from build123d import *

# Parameters (mm, degrees)
F0_R     = 4.838468
F0_W     = 33.466397
F0_H     = 30.935322
F0_R_2   = 5.460503
F1_DEPTH = 5.08


with BuildPart() as f1:
    # F0 (on Top) → F1 (new body)
    with BuildSketch(Plane.XY):
        with BuildLine():
            ThreePointArc((17.891966, -1.952547), (32.435058, 11.67451), (37.801563, 30.868229))
            ThreePointArc((37.801563, 30.868229), (-18.093211, 62.692563), (-16.933151, -1.616599))
            Line((-16.933151, -1.616599), (17.891966, -1.952547))
        make_face()
        with Locations((-12.703, 51.397717)):
            Circle(F0_R, mode=Mode.SUBTRACT)
        with Locations((1.265535, 25.170104)):
            Rectangle(F0_W, F0_H, mode=Mode.SUBTRACT)
        with Locations((13.170184, 51.397717)):
            Circle(F0_R_2, mode=Mode.SUBTRACT)
        with BuildLine():
            ThreePointArc((-10.608257, -4.338439), (-13.834146, -3.124943), (-16.933151, -1.616599))
            Line((-16.933151, -1.616599), (-16.933151, -58.892032))
            Line((-16.933151, -58.892032), (-16.933151, -60.651779))
            Line((-16.933151, -60.651779), (17.891966, -60.651779))
            Line((17.891966, -60.651779), (17.891966, -1.952547))
            ThreePointArc((17.891966, -1.952547), (15.052123, -3.282136), (12.109917, -4.366543))
            Line((12.109917, -4.366543), (12.109917, -56.126706))
            Line((12.109917, -56.126706), (-10.608257, -56.126706))
            Line((-10.608257, -56.126706), (-10.608257, -50.480825))
            Line((-10.608257, -50.480825), (-10.608257, -4.338439))
        make_face()
        with BuildLine():
            Line((17.891966, -1.952547), (-16.933151, -1.616599))
            ThreePointArc((-16.933151, -1.616599), (-13.834146, -3.124943), (-10.608257, -4.338439))
            ThreePointArc((-10.608257, -4.338439), (-7.87319, -5.109583), (-5.087015, -5.668589))
            ThreePointArc((-5.087015, -5.668589), (0.33248, -6.136051), (5.761954, -5.804015))
            ThreePointArc((5.761954, -5.804015), (8.967599, -5.225107), (12.109917, -4.366543))
            ThreePointArc((12.109917, -4.366543), (15.052123, -3.282136), (17.891966, -1.952547))
        make_face()
        with BuildLine():
            ThreePointArc((5.761954, -5.804015), (0.33248, -6.136051), (-5.087015, -5.668589))
            Line((-5.087015, -5.668589), (-5.087015, -50.480825))
            Line((-5.087015, -50.480825), (5.761954, -50.64771))
            Line((5.761954, -50.64771), (5.761954, -5.804015))
        make_face()
    extrude(amount=F1_DEPTH)


solid = f1.part
Work out the finished part from the listing and answer in its coordinate system (mm). A direction names the side the tool comes from. Give positions to 0.01 mm unless a question says otherwise; leave off trailing zeros. Loops run counter-clockwise (first coordinate to the right, second up) from the corner with the lowest first, then second, coordinate; pieces in that order, holes last. Notation, with made-up numbers: (8, 89.25) -> (36, 89.25) arc R17 cw to (36, 118.25) -> close; hole circle Ø2 at (14, 39.5). An arc over 180 degrees is marked (long way). Use a Markdown table: item, result. Add a question column.
1. Determine the mould class of faces 3 (the flat face through (17.892, -32, 3)), 4 (the flat face through (0, -60.652, 3)), 5 (the cylindrical face through (-13.3, 56.2, 2.5)) for opening direction Y: released by +Y, released by -Y, zero draft, split by the parting line, or undercut.
2. For faces 1 (the flat face through (-15.468, 25, 3)), 2 (the flat face through (0, 5, 5.08)), determine the directions among +Z, -Z, +X, -X, +Y, -Y from which every point of the face is accessible in a straight line to the end or side of a thin tool.
3. Find the intervals of material crossed by probe 1 along X at (y, z) = (-19, 4.15); probe 2 along X at (y, z) = (55.5, 0.4); probe 3 along Y at (x, z) = (2.5, 4.7), in increasing order.
4. Section D-D on y = 16 is taken. Determine the outline of the cut face in (x, z).
5. Section C-C on z = 1.95 is taken. Determine the outline of the cut face in (x, y), and give its area (3 significant figures).
6. Section A-A on y = -12 is taken. Determine the outline of the cut face in (x, z).
7. Section B-B on x = -13.5 is taken. Determine the outline of the cut face in (y, z).
8. Flat-ended cylindrical pins translate along their axes: pin 1 Ø1.5 at (x, z) = (-1.5, 4) entering from +Y; pin 2 Ø1.5 at (y, z) = (-29.5, 3.5) entering from -X; pin 3 Ø1.5 at (y, z) = (-27.5, 2) entering from +X. Find the tip coordinate at first contact, or state that the pin passes through.
Results below:
| question | item | result |
|---|---|---|
| 1 | face 3 | zero draft |
| 1 | face 4 | released by -Y |
| 1 | face 5 | undercut |
| 2 | face 1 | +Z, -Z |
| 2 | face 2 | +Z, +X, -X, +Y, -Y |
| 3 | probe 1 | x = -16.93 to -10.61, -5.09 to 5.76, 12.11 to 17.89 |
| 3 | probe 2 | x = -26.82 to -15.27, -10.14 to 9.57, 16.77 to 28.41 |
| 3 | probe 3 | y = -60.65 to -56.13, -50.6 to 9.7, 40.64 to 67.84 |
| 4 | outline | (-33.09, 0) -> (-15.47, 0) -> (-15.47, 5.08) -> (-33.09, 5.08) -> close; (18, 0) -> (34.68, 0) -> (34.68, 5.08) -> (18, 5.08) -> close |
| 5 | outline | (-16.93, -60.65) -> (17.89, -60.65) -> (17.89, -1.95) arc R37.01 ccw to (37.8, 30.87) arc R37.01 ccw (long way) to (-16.93, -1.62) -> close; hole circle Ø9.68 at (-12.7, 51.4); hole (-15.47, 9.7) -> (18, 9.7) -> (18, 40.64) -> (-15.47, 40.64) -> close; hole (-10.61, -56.13) -> (12.11, -56.13) -> (12.11, -4.37) arc R37.01 cw to (5.76, -5.8) -> (5.76, -50.65) -> (-5.09, -50.48) -> (-5.09, -5.67) arc R37.01 cw to (-10.61, -4.34) -> close; hole circle Ø10.92 at (13.17, 51.4) |
| 5 | area | 4,380 mm^2 |
| 6 | outline | (-16.93, 0) -> (-10.61, 0) -> (-10.61, 5.08) -> (-16.93, 5.08) -> close; (-5.09, 0) -> (5.76, 0) -> (5.76, 5.08) -> (-5.09, 5.08) -> close; (12.11, 0) -> (17.89, 0) -> (17.89, 5.08) -> (12.11, 5.08) -> close |
| 7 | outline | (-60.65, 0) -> (9.7, 0) -> (9.7, 5.08) -> (-60.65, 5.08) -> close; (40.64, 0) -> (46.63, 0) -> (46.63, 5.08) -> (40.64, 5.08) -> close; (56.17, 0) -> (65, 0) -> (65, 5.08) -> (56.17, 5.08) -> close |
| 8 | pin 1 | stops at y = 67.84 |
| 8 | pin 2 | stops at x = -16.93 |
| 8 | pin 3 | stops at x = 17.89 |
